```python
from build123d import *

# Parameters (mm, degrees)
SKETCH1_W               = 41
SKETCH1_H               = 93
BOSS_EXTRUDE1_DEPTH     = 42
CUT_EXTRUDE1_DEPTH      = 66.927991021
CUT_EXTRUDE1_DEPTH_BACK = 66.927991021
SKETCH2_R               = 1.125
CUT_EXTRUDE2_DEPTH      = 66.927991021
FILLET1_R               = 3
FILLET2_R               = 3


with BuildPart() as part:
    # Sketch1 → Boss-Extrude1 (new body)
    with BuildSketch(Plane(origin=(0, 0, 0), x_dir=(1, 0, 0), z_dir=(0, 1, 0))):
        Rectangle(SKETCH1_W, SKETCH1_H)
    extrude(amount=BOSS_EXTRUDE1_DEPTH)

    # Sketch2 → Cut-Extrude1 (cut, two sides: drawn at the far end of the back side and taken through both)
    with BuildSketch(Plane(origin=(0, 0, 0), x_dir=(-0.403397958441935, 0, 0.9150246374414619), z_dir=(-0.9150246374414619, 0, -0.403397958441935)).offset(-CUT_EXTRUDE1_DEPTH_BACK)):
        with Locations((-48.818303789, 40)):
            Circle(SKETCH2_R)
        with Locations((-48.818303789, 37.285714286)):
            Circle(SKETCH2_R)
        with Locations((-48.818303789, 34.571428571)):
            Circle(SKETCH2_R)
        with Locations((-48.818303789, 31.857142857)):
            Circle(SKETCH2_R)
        with Locations((-48.818303789, 29.142857143)):
            Circle(SKETCH2_R)
        with Locations((-48.818303789, 26.428571429)):
            Circle(SKETCH2_R)
        with Locations((-48.818303789, 23.714285714)):
            Circle(SKETCH2_R)
        with Locations((-48.818303789, 21)):
            Circle(SKETCH2_R)
        with Locations((-48.818303789, 18.285714286)):
            Circle(SKETCH2_R)
        with Locations((-48.818303789, 15.571428571)):
            Circle(SKETCH2_R)
        with Locations((-48.818303789, 12.857142857)):
            Circle(SKETCH2_R)
        with Locations((-48.818303789, 10.142857143)):
            Circle(SKETCH2_R)
        with Locations((-48.818303789, 7.428571429)):
            Circle(SKETCH2_R)
        with Locations((-48.818303789, 4.714285714)):
            Circle(SKETCH2_R)
        with Locations((-48.818303789, 2)):
            Circle(SKETCH2_R)
    extrude(amount=CUT_EXTRUDE1_DEPTH + CUT_EXTRUDE1_DEPTH_BACK, mode=Mode.SUBTRACT)

    # Sketch3 → Cut-Extrude2 (cut, through all)
    with BuildSketch(Plane.XZ):
        Polygon((16.5, 42.5), (-16.550825643, 42.5), (16.5, -32.468945972), align=None)
        Polygon((-16.5, 32.468945972), (16.550825643, -42.5), (-16.5, -42.5), align=None)
    extrude(amount=-CUT_EXTRUDE2_DEPTH, mode=Mode.SUBTRACT)

    # Fillet1
    fillet1_edges = [part.edges().sort_by_distance(p)[0] for p in [
        (-16.5, 21, -42.5),
        (-16.5, 21, 32.468945972),
        (16.550825643, 21, -42.5),
        (16.5, 21, 42.5),
        (16.5, 21, -32.468945972),
        (-16.550825643, 21, 42.5),
    ]]
    fillet(fillet1_edges, radius=FILLET1_R)

    # Fillet2
    fillet2_edges = [part.edges().sort_by_distance(p)[0] for p in [
        (-20.5, 21, 46.5),
    ]]
    fillet(fillet2_edges, radius=FILLET2_R)


solid = part.part
```
The model under review builds one solid part; all positions refer to its coordinate system, in mm. A direction names the side the tool comes from. Coordinates: 2 decimals unless noted, no trailing zeros. Write each loop counter-clockwise with the first axis right and the second up, starting at its lowest first coordinate (ties: lowest second). Pieces come first, ordered by that corner, then holes. Notation, with made-up numbers: (-32, 76.25) - (8, 76.25) arc R15 cw to (8, 82.25) - close; hole circle Ø4 at (22.5, -27). An arc over 180 degrees is marked (long way). Answer in a Markdown table with one row per item. Add a question column.
Q1. To check wall thickness, follow line 1 along Z through (x, y) = (-11.5, 12); line 2 along X through (y, z) = (25, -11); line 3 along Z through (x, y) = (-4.5, 30.5). State the ranges of each line that lie inside material, in increasing order. Write a range as from..to.
Q2. Consider section C-C on x = 3. Give the boundary of the cut face in (y, z).
Q3. Consider section D-D on z = 33. Give the boundary of the cut face in (x, y), then the cut area to 3 significant figures.
Q4. Consider section B-B on z = -30. Give the boundary of the cut face in (x, y).
Q5. For faces 4 (the face through (-14.062, 21.294, 21.174)), 5 (the face through (-19.64, 21.29, 45.6)), list the 3-axis set-ups (+Z, -Z, +X, -X, +Y, -Y) from which the entire face can be reached by the end or side of a thin tool; tool diameter is ignored.
Q6. Draft analysis for pull direction Y (two halves, no side actions). For faces 1 (the face through (-2, 42, 0)), 2 (the face through (17.576, 28.712, -44.468)), 3 (the face through (16.5, 21, 10)), state which applies: +Y half, -Y half, draft (parallel to the pull), parting line (faces both ways), or undercut.
Q7. Consider section A-A on z = 8. Give the boundary of the cut face in (x, y).
Answers below:
| question | item | result |
|---|---|---|
| 1 | line 1 | -46.5..-42.5, 20.46..31.04, 42.5..46.5 |
| 1 | line 2 | -20.5..-16.5, 2.66..7.04, 16.5..20.5 |
| 1 | line 3 | -46.5..-42.5, 5.25..15.17, 42.5..46.5 |
| 2 | outline | (0, -46.5) - (42, -46.5) - (42, -42.5) - (0, -42.5) - close; (0, -11.76) - (42, -11.76) - (42, -1.85) - (0, -1.85) - close; (0, 42.5) - (42, 42.5) - (42, 46.5) - (0, 46.5) - close |
| 3 | outline | (-20.5, 0) - (-12.36, 0) - (-12.36, 42) - (-20.5, 42) - close; (16.5, 0) - (20.5, 0) - (20.5, 42) - (16.5, 42) - close |
| 3 | area | 510 mm² |
| 4 | outline | (-20.5, 0) - (-16.5, 0) - (-16.5, 42) - (-20.5, 42) - close; (11.04, 0) - (20.5, 0) - (20.5, 42) - (11.04, 42) - close |
| 5 | face 4 | +Y, -Y |
| 5 | face 5 | +Z, -X, +Y, -Y |
| 6 | face 1 | +Y half |
| 6 | face 2 | undercut |
| 6 | face 3 | draft |
| 7 | outline | (-20.5, 0) - (-16.5, 0) - (-16.5, 42) - (-20.5, 42) - close; (-5.71, 0) - (-1.34, 0) - (-1.34, 42) - (-5.71, 42) - close; (16.5, 0) - (20.5, 0) - (20.5, 42) - (16.5, 42) - close |
